Geometry: see drawing. Coordinates: mm, zero at the bounding-box minimum. A direction names the side the tool comes from. Give positions to 0.01 mm unless a question says otherwise; leave off trailing zeros. Write each loop counter-clockwise with the first axis right and the second up, starting at its lowest first coordinate (ties: lowest second). Pieces come first, ordered by that corner, then holes. Notation, with made-up numbers: (-7.5, 73) - (33.5, 73) arc R21 ccw to (33.5, 97) - close; hole circle Ø6 at (34, 38). An arc over 180 degrees is marked (long way). One line per question, with ' | ' between items. Start each with the question number.
(1) Ray query, line 1 (Y direction, x = 133, z = 15); line 2 (X direction, y = 17, z = 25.5); line 3 (Z direction, x = 65.5, y = 15.25). Return the intervals inside material, ascending. Write a range as [from, to].
(2) Section A-A, the plane z = 54.5. Return loops of the section in (x, y).
(3) Access query for the marked faces 1, 2, 3, 4 and 5. Directions: +Z, -Z, +X, -X, +Y, -Y. A direction counts if a zero-diameter tool reaches every point of the face in a straight line with its end or side. Return the directions, or none.
(4) Section C-C, the plane x = 59. Return loops of the section in (y, z) (1 decimal), plus the area to 3 significant figures.
(5) Section B-B, the plane y = 6.5. Return loops of the section in (x, z) (1 decimal), plus the area to 3 significant figures.
(6) Pin query (flat end, axial travel): pin 1 (10 mm diameter, centred on x = 60, y = 14.5, fed in from +Z); pin 2 (3 mm diameter, centred on x = 90, y = 16.5, fed in from -Z); pin 3 (3 mm diameter, centred on y = 18, z = 40, fed in from +X); pin 4 (5 mm diameter, centred on x = 6, z = 55.5, fed in from -Y). Return the tip coordinate at first contact, or that it passes through.
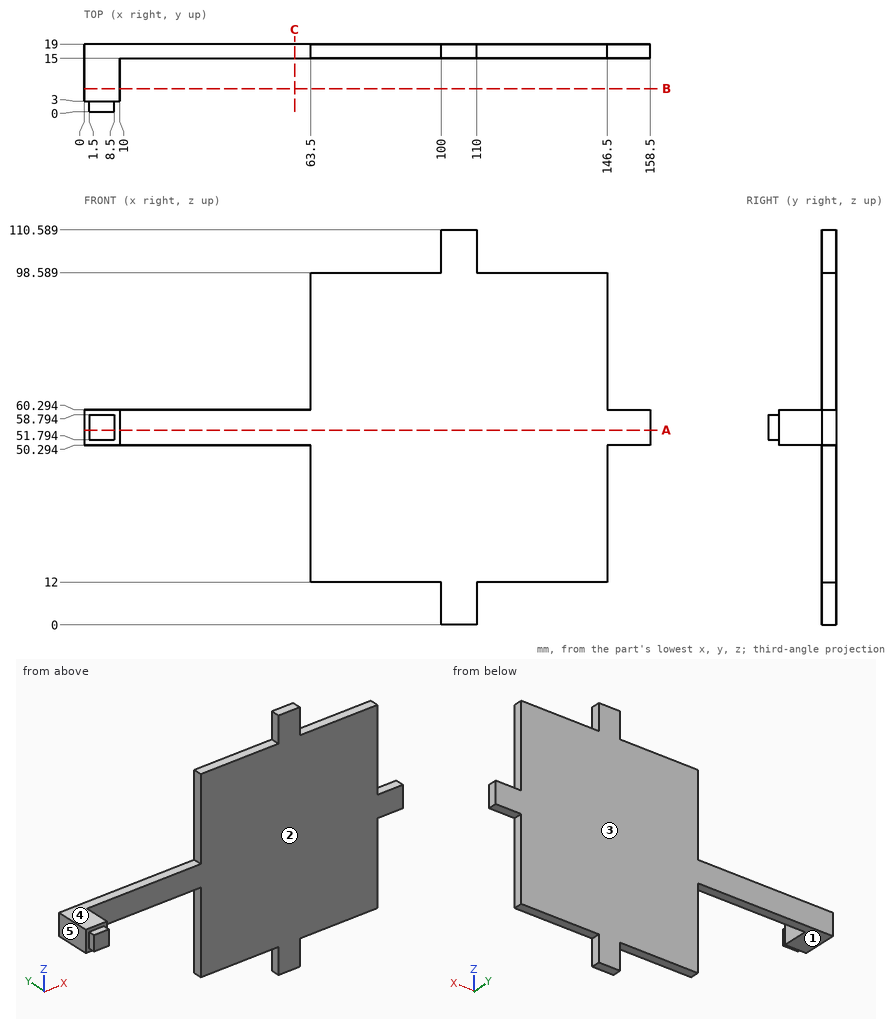
Check sheet entries:
1) line 1: [15, 19] | line 2: [63.5, 146.5] | line 3: [12, 98.59]
2) outline: (0, 3) - (1.5, 3) - (1.5, 0) - (8.5, 0) - (8.5, 3) - (10, 3) - (10, 15) - (158.5, 15) - (158.5, 19) - (0, 19) - close
3) face 1: -Z, -X, +Y, -Y | face 2: +Z, -Z, +X, -Y | face 3: +Z, -Z, +X, -X, +Y | face 4: +Z, -X, +Y, -Y | face 5: +Z, -Z, -X, +Y, -Y
4) outline: (15, 50.3) - (19, 50.3) - (19, 60.3) - (15, 60.3) - close | area: 40.0 mm²
5) outline: (0, 50.3) - (10, 50.3) - (10, 60.3) - (0, 60.3) - close | area: 100 mm²
6) pin 1: z = 98.59 | pin 2: z = 12 | pin 3: x = 146.5 | pin 4: y = 0
